from build123d import *

# Parameters (mm, degrees)
BOX095_W     = 3
BOX095_H     = 32
BOX095_DEPTH = 42
BOX094_W     = 3
BOX094_H     = 32
BOX094_DEPTH = 42
BOX093_W     = 3
BOX093_H     = 32
BOX093_DEPTH = 42
BOX092_W     = 3
BOX092_H     = 32
BOX092_DEPTH = 42
BOX091_W     = 3
BOX091_H     = 18
BOX091_DEPTH = 24


with BuildPart() as box095:
    # Box095 → Box095 (new body)
    with BuildSketch(Plane(origin=(99, 8, 67), x_dir=(1, 0, 0), z_dir=(0, 0, 1))):
        with Locations((1.5, 16)):
            Rectangle(BOX095_W, BOX095_H)
    extrude(amount=BOX095_DEPTH)


with BuildPart() as box094:
    # Box094 → Box094 (new body)
    with BuildSketch(Plane(origin=(141, 8, 109), x_dir=(0, 0, 1), z_dir=(-1, 0, 0))):
        with Locations((1.5, 16)):
            Rectangle(BOX094_W, BOX094_H)
    extrude(amount=BOX094_DEPTH)


with BuildPart() as box093:
    # Box093 → Box093 (new body)
    with BuildSketch(Plane(origin=(138, 8, 67), x_dir=(1, 0, 0), z_dir=(0, 0, 1))):
        with Locations((1.5, 16)):
            Rectangle(BOX093_W, BOX093_H)
    extrude(amount=BOX093_DEPTH)


with BuildPart() as box092:
    # Box092 → Box092 (new body)
    with BuildSketch(Plane(origin=(141, 8, 64), x_dir=(0, 0, 1), z_dir=(-1, 0, 0))):
        with Locations((1.5, 16)):
            Rectangle(BOX092_W, BOX092_H)
    extrude(amount=BOX092_DEPTH)


with BuildPart() as fusion117:
    # Box091 → Box091 (new body)
    with BuildSketch(Plane(origin=(99, -10, 80), x_dir=(1, 0, 0), z_dir=(0, 0, 1))):
        with Locations((1.5, 9)):
            Rectangle(BOX091_W, BOX091_H)
    extrude(amount=BOX091_DEPTH)

    # Fusion117: union Box095, Box094, Box093, Box092
    add(box095.part)
    add(box094.part)
    add(box093.part)
    add(box092.part)


solid = fusion117.part
Can you work these out from the model? Positions are in its coordinate system, mm. A direction names the side the tool comes from. Give positions to 0.01 mm unless a question says otherwise; leave off trailing zeros. Loops run counter-clockwise (first coordinate to the right, second up) from the corner with the lowest first, then second, coordinate; pieces in that order, holes last. Notation, with made-up numbers: (64.25, 55) -> (113.25, 55) arc R24 cw to (113.25, 78) -> close; hole circle Ø7 at (-14.75, -33.5). An arc over 180 degrees is marked (long way). Use one line per item in the form item = value.
1) If we section it at B-B (x = 106): Please give me the cut outline in (y, z), plus the area to 3 significant figures.
Answers:
outline = (8, 64) -> (40, 64) -> (40, 67) -> (8, 67) -> close; (8, 109) -> (40, 109) -> (40, 112) -> (8, 112) -> close
area = 192 mm²
2) I need wall thicknesses on line 1 along Z through (x, y) = (126, 11.5); line 2 along X through (y, z) = (37.5, 86); line 3 along X through (y, z) = (1.5, 91.5). Which ranges of each line are inside material? Lowest first, please.
Answers:
line_1 = 64 to 67, 109 to 112
line_2 = 99 to 102, 138 to 141
line_3 = 99 to 102
3) If we section it at D-D (y = -6): Please give me the cut outline in (x, z), plus the area to 3 significant figures.
Answers:
outline = (99, 80) -> (102, 80) -> (102, 104) -> (99, 104) -> close
area = 72.0 mm²
4) If we section it at A-A (y = 28): Please give me the cut outline in (x, z).
Answers:
outline = (99, 64) -> (141, 64) -> (141, 112) -> (99, 112) -> close; hole (102, 67) -> (138, 67) -> (138, 109) -> (102, 109) -> close
5) For faces 4 (the face through (102, 20, 88)), 5 (the face through (100, -1, 80)), 6 (the face through (141, 24, 88)), which set-ups out of +Z, -Z, +X, -X, +Y, -Y let a thin tool reach every point of the face, with its end or its side?
Answers:
face_4 = +Y, -Y
face_5 = -Z, +X, -X, -Y
face_6 = +Z, -Z, +X, +Y, -Y
6) Will these pins go through, and if not, where does the flat tip stop? pin 1 (6 mm diameter, centred on y = 2, z = 83, fed in from +X); pin 2 (12 mm diameter, centred on x = 133, y = -1.5, fed in from -Z); pin 3 (3.5 mm diameter, centred on x = 100, y = 0, fed in from +Z); pin 4 (0.9 mm diameter, centred on x = 101, y = -4, fed in from -Z).
Answers:
pin_1 = 102
pin_2 = through
pin_3 = 104
pin_4 = 80
7) If we section it at C-C (z = 88): Please give me the cut outline in (x, y).
Answers:
outline = (99, -10) -> (102, -10) -> (102, 40) -> (99, 40) -> close; (138, 8) -> (141, 8) -> (141, 40) -> (138, 40) -> close
8) We'd pull the mould along X, two halves only. Please class faces 1 (the face through (120, 24, 67)), 2 (the face through (100, -1, 104)), 3 (the face through (99, 21, 88)): released by +X, released by -X, zero draft, split by the parting line, or undercut.
Answers:
face_1 = undercut
face_2 = zero draft
face_3 = released by -X
